Source: CAD feature listing. Evaluate the final solid. Frame: model axes, mm. Face numbers are marked on the shaded views. A direction names the side the tool comes from. Give positions to 0.01 mm unless a question says otherwise; leave off trailing zeros. Write each loop counter-clockwise with the first axis right and the second up, starting at its lowest first coordinate (ties: lowest second). Pieces come first, ordered by that corner, then holes. Notation, with made-up numbers: (-30.75, 43) -> (-19.75, 43) arc R14 cw to (-19.75, 50) -> close; hole circle Ø6 at (23.25, -2.5). An arc over 180 degrees is marked (long way). Write item = value, one per line.
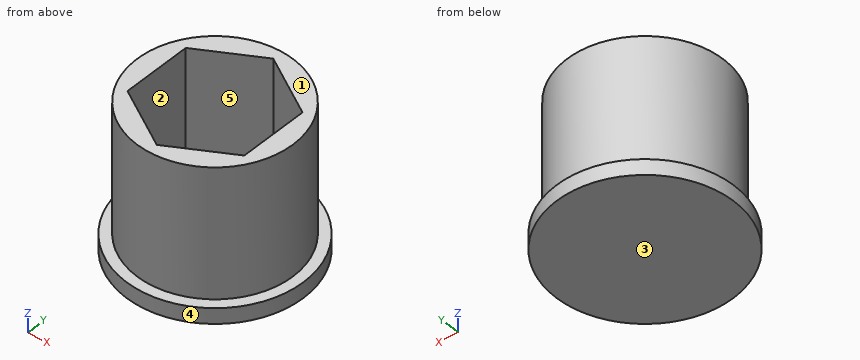
from build123d import *

# Parameters (mm, degrees)
SKETCH_R     = 17
PAD_DEPTH    = 3
SKETCH001_R  = 14.990381
PAD001_DEPTH = 25


with BuildPart() as part:
    # Sketch → Pad (new body)
    with BuildSketch(Plane.XY):
        Circle(SKETCH_R)
    extrude(amount=PAD_DEPTH)

    # Sketch001 (on Face3 of Pad) → Pad001 (join)
    with BuildSketch(Plane.XY.offset(3)):
        Circle(SKETCH001_R)
        Polygon((-11.25, 6.495191), (-11.25, -6.495191), (0, -12.990381), (11.25, -6.495191), (11.25, 6.495191), (0, 12.990381), align=None, mode=Mode.SUBTRACT)
    extrude(amount=PAD001_DEPTH)


solid = part.part
(1) Section query A-A (z = 19). Return loops of the section in (x, y).
Values follow:
outline = circle Ø29.98 at (0, 0); hole (-11.25, -6.5) -> (0, -12.99) -> (11.25, -6.5) -> (11.25, 6.5) -> (0, 12.99) -> (-11.25, 6.5) -> close
(2) Pull-direction query (Y, two-part tool) for the marked faces 3, 4 and 5; classes: pulls with the +Y half, pulls with the -Y half, needs draft (parallel to the pull), parting line crosses it, or undercut.
Values follow:
face_3 = needs draft
face_4 = parting line crosses it
face_5 = undercut
(3) Access query for the marked faces 1 and 2. Directions: +Z, -Z, +X, -X, +Y, -Y. A direction counts if a zero-diameter tool reaches every point of the face in a straight line with its end or side. Return the directions, or none.
Values follow:
face_1 = +Z, +X, -X, +Y, -Y
face_2 = +Z
(4) Section query D-D (y = -8.5). Return loops of the section in (x, z), plus the area to 3 significant figures.
Values follow:
outline = (-14.72, 0) -> (14.72, 0) -> (14.72, 3) -> (12.35, 3) -> (12.35, 28) -> (7.78, 28) -> (7.78, 3) -> (-7.78, 3) -> (-7.78, 28) -> (-12.35, 28) -> (-12.35, 3) -> (-14.72, 3) -> close
area = 317 mm2
(5) Section query B-B (y = 0). Return loops of the section in (x, z), plus the area to 3 significant figures.
Values follow:
outline = (-17, 0) -> (17, 0) -> (17, 3) -> (14.99, 3) -> (14.99, 28) -> (11.25, 28) -> (11.25, 3) -> (-11.25, 3) -> (-11.25, 28) -> (-14.99, 28) -> (-14.99, 3) -> (-17, 3) -> close
area = 289 mm2
(6) Material intervals for line 1 (Z direction, x = -9, y = 6.5); line 2 (X direction, y = 3, z = 11.5); line 3 (X direction, y = -10.5, z = 4), sorted ascending.
Values follow:
line_1 = 0 to 3
line_2 = -14.69 to -11.25, 11.25 to 14.69
line_3 = -10.7 to -4.31, 4.31 to 10.7
(7) First-contact query: pin 1 (8 mm diameter, centred on y = 9.5, z = 22.5, fed in from -X); pin 2 (6.5 mm diameter, centred on y = 1, z = 18, fed in from +X); pin 3 (8 mm diameter, centred on x = 6, z = 16, fed in from -Y). Flat tips, straight axial feed; report the tip coordinate or a pass-through.
Values follow:
pin_1 = -13.94
pin_2 = 14.99
pin_3 = -14.86
(8) Section query C-C (x = 12.5). Return loops of the section in (y, z), plus the area to 3 significant figures.
Values follow:
outline = (-11.52, 0) -> (11.52, 0) -> (11.52, 3) -> (8.27, 3) -> (8.27, 28) -> (-8.27, 28) -> (-8.27, 3) -> (-11.52, 3) -> close
area = 483 mm2
